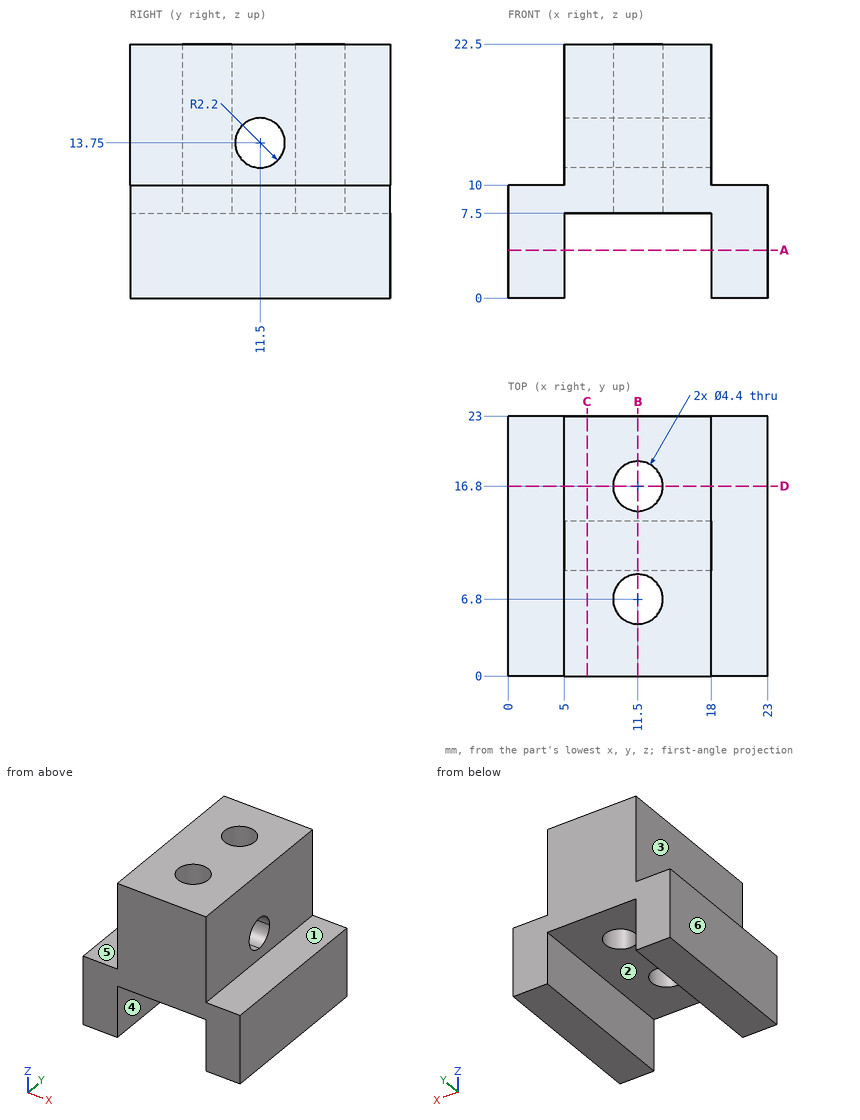
Part print with two shaded views. Sizes in mm from the minimum x, y, z corner. A direction names the side the tool comes from. Round coordinates to 2 decimals unless told otherwise and drop trailing zeros. Loops run counter-clockwise (first coordinate to the right, second up) from the corner with the lowest first, then second, coordinate; pieces in that order, holes last.
Item 1: Two-plate mould, pull along X, no slides. Class the marked faces 4, 5 and 6: released by +X, released by -X, zero draft, split by the parting line, or undercut.
Item 2: Which spindle directions (+Z, -Z, +X, -X, +Y, -Y) get a long thin tool onto all of the face, cutting with end or side? Do the marked faces 1, 2 and 3. Say none if no direction does.
Item 3: Saw through at D-D (y = 16.8). List the corners of the cut face in (x, z).
Item 4: Saw through at C-C (x = 7). List the corners of the cut face in (y, z).
Item 5: Saw through at B-B (x = 11.5). List the corners of the cut face in (y, z), then the cut area to 3 significant figures.
Item 6: Saw through at A-A (z = 4.25). List the corners of the cut face in (x, y).
Item 7: Pin check, flat tips, straight feed: P1, Ø2, axis at x = 12, y = 13, coming from the -Z side; P2, Ø4, axis at y = 6, z = 17.5, coming from the -X side; P3, Ø1.5, axis at x = 19.5, y = 13.5, coming from the +Z side. Stop position of each tip, or through.
Item 8: Drill centre lines: line 1 along Y through (x, z) = (11.5, 17.5); line 2 along X through (y, z) = (5.25, 5.25); line 3 along Y through (x, z) = (9.5, 18.75). Where is each one in solid material? Low to high.
Worked answers:
1. face 4: undercut
1. face 5: zero draft
1. face 6: released by -X
2. face 1: +Z, +X, +Y, -Y
2. face 2: -Z, +Y, -Y
2. face 3: +Z, -X, +Y, -Y
3. outline: (0, 0) - (5, 0) - (5, 7.5) - (9.3, 7.5) - (9.3, 22.5) - (5, 22.5) - (5, 10) - (0, 10) - close; (13.7, 7.5) - (18, 7.5) - (18, 0) - (23, 0) - (23, 10) - (18, 10) - (18, 22.5) - (13.7, 22.5) - close
4. outline: (0, 7.5) - (23, 7.5) - (23, 22.5) - (0, 22.5) - close; hole circle Ø4.4 at (11.5, 13.75)
5. outline: (0, 7.5) - (4.6, 7.5) - (4.6, 22.5) - (0, 22.5) - close; (9, 7.5) - (14.6, 7.5) - (14.6, 22.5) - (9, 22.5) - close; (19, 7.5) - (23, 7.5) - (23, 22.5) - (19, 22.5) - close; hole circle Ø4.4 at (11.5, 13.75)
5. area: 198 mm2
6. outline: (0, 0) - (5, 0) - (5, 23) - (0, 23) - close; (18, 0) - (23, 0) - (23, 23) - (18, 23) - close
7. P1: stops at z = 7.5
7. P2: stops at x = 5
7. P3: stops at z = 10
8. line 1: y = 0 to 4.6, 9 to 14.6, 19 to 23
8. line 2: x = 0 to 5, 18 to 23
8. line 3: y = 0 to 5.88, 7.72 to 15.88, 17.72 to 23
